For this review, take the finished solid that the model builds, in its own axes (mm). A direction names the side the tool comes from. Coordinates: 2 decimals unless noted, no trailing zeros. Order: outer loops, then holes, each group sorted by start corner. A loop starts at its lowest first (then second) coordinate and runs counter-clockwise, first axis right, second up. Notation, with made-up numbers: (12.5, 51) -> (70.5, 51) arc R17 ccw to (70.5, 72) -> close; hole circle Ø10 at (4.25, 70). An arc over 180 degrees is marked (long way). Answer as a JSON object with one key per item and string values. Group by question number.
1) For pin 1 (2 mm diameter, centred on x = 7.5, z = 18, fed in from -Y); pin 2 (24.5 mm diameter, centred on x = 4.82, z = 9.78, fed in from -Y), all flat-tipped, find the tip position at first contact; note any pin that passes through.
2) Add section A-A, the plane x = 9. Write out the cut boundary in (y, z), then the cut area to 3 significant figures.
3) Add section C-C, the plane y = -66. Write out the cut boundary in (x, z), then the cut area to 3 significant figures.
4) Draft analysis for pull direction X (two halves, no side actions). For faces 1 (the flat face through (-10, -101.6, 4)), 2 (the cylindrical face through (3.323, -25.044, 21.166)), 3 (the flat face through (-26.719, -50, 8)), state which applies: +X half, -X half, draft (parallel to the pull), parting line (faces both ways), or undercut.
5) Wall thickness on L1, parallel to X at y = -59, z = 10.5; L2, parallel to Y at x = 18, z = 8; L3, parallel to X at y = -74.5, z = 24: over which ranges is each line inside the solid? List them lowest first.
6) Add section B-B, the plane z = 7.5. Write out the cut boundary in (x, y).
7) Add section D-D, the plane z = -3. Write out the cut boundary in (x, y).
8) Machinability: for faces 4 (the cylindrical face through (-6.505, -75.844, 20.165)), 5 (the flat face through (-3, 0, -1)), which of the approach directions +Z, -Z, +X, -X, +Y, -Y give a long, thin tool a straight path to every point of the face, cutting with its end or side? Answer none if there is none.
from build123d import *

# Parameters (mm, degrees)
F0_W     = 61.6135448217
F0_H     = 45.5531394109
F0_R     = 15.3630255382
F0_R_2   = 11.4814952194
F1_DEPTH = 50.8
F2_DEPTH = 101.6


# Not quite as in the source:
# - the program builds the solid bodies; features that only make, move or delete a surface that nothing else refers to are left out


with BuildPart() as f1:
    # F0 (on Front) → F1 (new body)
    with BuildSketch(Plane.XZ):
        with Locations((4.0881037712, 8.3222077228)):
            Rectangle(F0_W, F0_H)
        with Locations((4.818121437, 9.7822444513)):
            Circle(F0_R, mode=Mode.SUBTRACT)
        with Locations((4.818121437, 9.7822444513)):
            Circle(F0_R)
        with Locations((4.818121437, 9.7822444513)):
            Circle(F0_R_2, mode=Mode.SUBTRACT)
    extrude(amount=F1_DEPTH)

    # F0 (on Front) → F2 (join)
    with BuildSketch(Plane.XZ):
        with Locations((4.0881037712, 8.3222077228)):
            Rectangle(F0_W, F0_H)
        with Locations((4.818121437, 9.7822444513)):
            Circle(F0_R, mode=Mode.SUBTRACT)
    extrude(amount=F2_DEPTH)


solid = f1.part
Output values:
{
 "1": {"pin 1": "passes through", "pin 2": "stops at y = -50.8"},
 "2": {"outline": "(-101.6, -14.45) -> (0, -14.45) -> (0, -0.91) -> (-50.8, -0.91) -> (-50.8, -5) -> (-101.6, -5) -> close; (-101.6, 24.57) -> (-50.8, 24.57) -> (-50.8, 20.48) -> (0, 20.48) -> (0, 31.1) -> (-101.6, 31.1) -> close", "area": "2,040 mm²"},
 "3": {"outline": "(-26.72, -14.45) -> (34.89, -14.45) -> (34.89, 31.1) -> (-26.72, 31.1) -> close; hole circle Ø30.73 at (4.82, 9.78)", "area": "2,070 mm²"},
 "4": {"face 1": "draft", "face 2": "undercut", "face 3": "-X half"},
 "5": {"L1": "x = -26.72 to -10.53, 20.16 to 34.89", "L2": "y = -50.8 to 0", "L3": "x = -26.72 to -1, 10.64 to 34.89"},
 "6": {"outline": "(-26.72, -101.6) -> (-10.37, -101.6) -> (-10.37, -50.8) -> (-6.43, -50.8) -> (-6.43, 0) -> (-26.72, 0) -> close; (16.07, -50.8) -> (20.01, -50.8) -> (20.01, -101.6) -> (34.89, -101.6) -> (34.89, 0) -> (16.07, 0) -> close"},
 "7": {"outline": "(-26.72, -101.6) -> (-3.7, -101.6) -> (-3.7, -50.8) -> (13.34, -50.8) -> (13.34, -101.6) -> (34.89, -101.6) -> (34.89, 0) -> (-26.72, 0) -> close"},
 "8": {"face 4": "-Y", "face 5": "+Z, -Z, +X, -X, +Y"}
}
